```python
from build123d import *

# Parameters (mm, degrees)
BOSS_EXTRUDE1_DEPTH     = 3.5
BOSS_EXTRUDE2_DEPTH     = 7
SKETCH3_R               = 1.5
SKETCH3_W               = 8
SKETCH3_H               = 8
SKETCH3_R_2             = 2.5
BOSS_EXTRUDE3_DEPTH     = 4.5
SKETCH4_R               = 2.5
BOSS_EXTRUDE4_DEPTH     = 4.5
CUT_EXTRUDE1_DEPTH      = 123.693401635
CUT_EXTRUDE1_DEPTH_BACK = 123.693401635
SKETCH5_R               = 2.5
SKETCH5_R_2             = 2.55926668
SKETCH5_R_3             = 1.5
FILLET1_R               = 3.5


with BuildPart() as part:
    # Sketch1 → Boss-Extrude1 (new body)
    with BuildSketch(Plane(origin=(0, 0, 0), x_dir=(1, 0, 0), z_dir=(0, 1, 0))):
        Polygon((-57.597316241, 51.805869074), (-57.597316241, -8.444130926), (-46.097316241, -28.194130926), (-46.097316241, -108.194130926), (43.902683759, -108.194130926), (43.902683759, -28.194130926), (55.402683759, -8.444130926), (55.402683759, 51.805869074), align=None)
    extrude(amount=BOSS_EXTRUDE1_DEPTH)

    # Sketch2 → Boss-Extrude2 (add)
    with BuildSketch(Plane(origin=(0, 3.5, 0), x_dir=(1, 0, 0), z_dir=(0, 1, 0))):
        Polygon((-46.097316241, -28.194130926), (-46.097316241, -108.194130926), (43.902683759, -108.194130926), (43.902683759, -28.194130926), (41.402683759, -28.194130926), (41.402683759, -105.694130926), (-43.597316241, -105.694130926), (-43.597316241, -28.194130926), align=None)
        Polygon((52.902683759, -6.988434723), (55.402683759, -8.444130926), (43.902683759, -28.194130926), (41.402683759, -26.738434723), align=None)
        Polygon((41.402683759, -28.194130926), (43.902683759, -28.194130926), (41.402683759, -26.738434723), align=None)
        Polygon((52.902683759, -6.988434723), (55.402683759, -8.444130926), (55.402683759, -6.988434723), align=None)
        Polygon((-57.597316241, 51.805869074), (-57.597316241, -6.988434723), (-55.097316241, -6.988434723), (-55.097316241, 49.305869074), (52.902683759, 49.305869074), (52.902683759, -6.988434723), (55.402683759, -6.988434723), (55.402683759, 51.805869074), align=None)
        Polygon((-43.597316241, -26.738434723), (-46.097316241, -28.194130926), (-43.597316241, -28.194130926), align=None)
        Polygon((-43.597316241, -26.738434723), (-46.097316241, -28.194130926), (-57.597316241, -8.444130926), (-55.097316241, -6.988434723), align=None)
        Polygon((-57.597316241, -6.988434723), (-57.597316241, -8.444130926), (-55.097316241, -6.988434723), align=None)
    extrude(amount=BOSS_EXTRUDE2_DEPTH)

    # Sketch3 → Boss-Extrude3 (add)
    # profile 1 of 3: a face of its own
    with BuildSketch(Plane(origin=(0, 3.5, 0), x_dir=(1, 0, 0), z_dir=(0, 1, 0))):
        Polygon((-43.597316241, -99.694130926), (-43.597316241, -105.694130926), (41.402683759, -105.694130926), (41.402683759, -99.694130926), (32.902683759, -99.694130926), (20.902683759, -102.694130926), (-23.097316241, -102.694130926), (-35.097316241, -99.694130926), align=None)
        with Locations(Location((-39.347316241, -101.944130926, 0), (0, 0, 270))):
            Circle(SKETCH3_R, mode=Mode.SUBTRACT)
        with Locations(Location((37.152683759, -101.944130926, 0), (0, 0, 270))):
            Circle(SKETCH3_R, mode=Mode.SUBTRACT)
    # profile 2 of 3: a face of its own
    with BuildSketch(Plane(origin=(0, 3.5, 0), x_dir=(1, 0, 0), z_dir=(0, 1, 0))):
        with Locations((-51.097316241, 45.305869074)):
            Rectangle(SKETCH3_W, SKETCH3_H)
        with Locations(Location((-51.097316241, 45.305869074, 0), (0, 0, 270))):
            Circle(SKETCH3_R_2, mode=Mode.SUBTRACT)
    # profile 3 of 3: a face of its own
    with BuildSketch(Plane(origin=(0, 3.5, 0), x_dir=(1, 0, 0), z_dir=(0, 1, 0))):
        with Locations((48.902683759, 45.305869074)):
            Rectangle(SKETCH3_W, SKETCH3_H)
        with Locations(Location((48.902683759, 45.305869074, 0), (0, 0, 270))):
            Circle(SKETCH3_R_2, mode=Mode.SUBTRACT)
    extrude(amount=BOSS_EXTRUDE3_DEPTH)

    # Sketch4 → Boss-Extrude4 (add)
    # profile 1 of 2: a face of its own
    with BuildSketch(Plane(origin=(0, 3.5, 0), x_dir=(1, 0, 0), z_dir=(0, 1, 0))):
        Polygon((1.402683759, 10.130869074), (-55.097316241, 10.130869074), (-55.097316241, -6.988434723), (-43.597316241, -26.738434723), (-43.597316241, 0.130869074), (1.402683759, 0.130869074), align=None)
        with Locations(Location((-31.847316241, 5.130869074, 0), (0, 0, 90))):
            Circle(SKETCH4_R, mode=Mode.SUBTRACT)
        with Locations(Location((-21.847316241, 5.130869074, 0), (0, 0, 90))):
            Circle(SKETCH4_R, mode=Mode.SUBTRACT)
    # profile 2 of 2: a face of its own
    with BuildSketch(Plane(origin=(0, 3.5, 0), x_dir=(1, 0, 0), z_dir=(0, 1, 0))):
        Polygon((39.6145491, 10.130869074), (39.6145491, 0.130869074), (41.402683759, 0.130869074), (41.402683759, -26.738434723), (52.902683759, -6.988434723), (52.902683759, 10.130869074), align=None)
    extrude(amount=BOSS_EXTRUDE4_DEPTH)

    # Sketch5 → Cut-Extrude1 (cut, two sides: drawn at the far end of the back side and taken through both)
    with BuildSketch(Plane(origin=(0, 5, 0), x_dir=(1, 0, 0), z_dir=(0, 1, 0)).offset(-CUT_EXTRUDE1_DEPTH_BACK)):
        with Locations(Location((-21.847316241, 5.130869074, 0), (0, 0, 90))):
            Circle(SKETCH5_R)
        with Locations(Location((-31.847316241, 5.130869074, 0), (0, 0, 270))):
            Circle(SKETCH5_R_2)
        with Locations(Location((-39.347316241, -101.944130926, 0), (0, 0, 270))):
            Circle(SKETCH5_R_3)
        with Locations(Location((37.152683759, -101.944130926, 0), (0, 0, 270))):
            Circle(SKETCH5_R_3)
        with Locations(Location((-51.097316241, 45.305869074, 0), (0, 0, 270))):
            Circle(SKETCH5_R)
        with Locations(Location((48.902683759, 45.305869074, 0), (0, 0, 270))):
            Circle(SKETCH5_R)
        with Locations(Location((-49.597316241, -6.988434723, 0), (0, 0, 270))):
            Circle(SKETCH5_R)
        with Locations(Location((47.402683759, -6.988434723, 0), (0, 0, 270))):
            Circle(SKETCH5_R)
    extrude(amount=CUT_EXTRUDE1_DEPTH + CUT_EXTRUDE1_DEPTH_BACK, mode=Mode.SUBTRACT)

    # Fillet1
    # the kernel refuses this fillet: 3.5 mm, written as the material it adds along each edge
    with BuildSketch(Plane(origin=(41.402683759, 3.5, 99.694130926), x_dir=(0, 0, -1), z_dir=(0, 1, 0)), Plane(origin=(-43.597316241, 3.5, 99.694130926), x_dir=(1, 0, 0), z_dir=(0, 1, 0)), Plane(origin=(-55.097316241, 3.5, -41.305869074), x_dir=(0, 0, 1), z_dir=(0, 1, 0)), Plane(origin=(-47.097316241, 3.5, -49.305869074), x_dir=(0, 0, 1), z_dir=(0, 1, 0)), Plane(origin=(52.902683759, 3.5, -41.305869074), x_dir=(-1, 0, 0), z_dir=(0, 1, 0)), Plane(origin=(-55.097316241, 3.5, -10.130869074), x_dir=(1, 0, 0), z_dir=(0, 1, 0))) as fillet1_piece_1:
        with BuildLine():
            CenterArc((FILLET1_R, FILLET1_R), FILLET1_R, 180, 90)
            Line((0, FILLET1_R), (0, 0))
            Line((0, 0), (FILLET1_R, 0))
        make_face()
    extrude(amount=4.5)
    with BuildSketch(Plane(origin=(20.902683759, 2.422825776, 102.694130926), x_dir=(0.9701425001453338, 0, -0.2425356250363252), z_dir=(0, 1, 0)), Plane(origin=(-23.097316241, 2.422825776, 102.694130926), x_dir=(1, 0, 0), z_dir=(0, 1, 0))) as fillet1_piece_2:
        with BuildLine():
            CenterArc((FILLET1_R * 0.123105625618, FILLET1_R), FILLET1_R, 255.963756532, 14.036243468)
            Line((-FILLET1_R * 0.119429999419, FILLET1_R * 0.0298574998547), (0, 0))
            Line((0, 0), (FILLET1_R * 0.123105625618, 0))
        make_face()
    extrude(amount=5.577174224)
    with BuildSketch(Plane(origin=(44.902683759, 3.5, -49.305869074), x_dir=(0, 0, 1), z_dir=(0, 1, 0)), Plane(origin=(52.902683759, 3.5, -10.130869074), x_dir=(-1, 0, 0), z_dir=(0, 1, 0)), Plane(origin=(-43.597316241, 3.5, -0.130869074), x_dir=(1, 0, 0), z_dir=(0, 1, 0))) as fillet1_piece_3:
        with BuildLine():
            CenterArc((FILLET1_R, -FILLET1_R), FILLET1_R, 90, 90)
            Line((0, -FILLET1_R), (0, 0))
            Line((0, 0), (FILLET1_R, 0))
        make_face()
    extrude(amount=4.5)
    with BuildSketch(Plane(origin=(43.902683759, 10.5, 28.194130926), x_dir=(0, 0, 1), z_dir=(0, -1, 0)), Plane(origin=(-46.097316241, 0, 28.194130926), x_dir=(0, 0, 1), z_dir=(0, 1, 0))) as fillet1_piece_4:
        with BuildLine():
            CenterArc((FILLET1_R * 0.269926710528, -FILLET1_R), FILLET1_R, 90, 30.211322386)
            Line((-FILLET1_R * 0.23326401814, -FILLET1_R * 0.135824618157), (0, 0))
            Line((0, 0), (FILLET1_R * 0.269926710528, 0))
        make_face()
    extrude(amount=10.5)
    with BuildSketch(Plane(origin=(41.402683759, 3.5, -0.130869074), x_dir=(-1, 0, 0), z_dir=(0, 1, 0))) as fillet1_piece_5:
        with BuildLine():
            CenterArc((3.5, 3.052788407), FILLET1_R, 180, 60.718267745)
            Line((0, 3.052788407), (0, 0))
            Line((0, 0), (1.788134659, 0))
        make_face()
    extrude(amount=4.5)
    # the kernel refuses this fillet: 3.5 mm, written as the material it takes off along each edge
    with BuildSketch(Plane(origin=(32.902683759, 3.5, 99.694130926), x_dir=(-0.9701425001453338, 0, 0.2425356250363252), z_dir=(0, 1, 0)), Plane(origin=(-35.097316241, 3.5, 99.694130926), x_dir=(-1, 0, 0), z_dir=(0, 1, 0))) as fillet1_2_piece_1:
        with BuildLine():
            CenterArc((FILLET1_R * 0.123105625618, FILLET1_R), FILLET1_R, 255.963756532, 14.036243468)
            Line((-FILLET1_R * 0.119429999419, FILLET1_R * 0.0298574998547), (0, 0))
            Line((0, 0), (FILLET1_R * 0.123105625618, 0))
        make_face()
    extrude(amount=5.577174224, mode=Mode.SUBTRACT)
    with BuildSketch(Plane(origin=(-47.097316241, 3.5, -41.305869074), x_dir=(0, 0, -1), z_dir=(0, 1, 0)), Plane(origin=(44.902683759, 3.5, -41.305869074), x_dir=(1, 0, 0), z_dir=(0, 1, 0)), Plane(origin=(39.6145491, 3.5, -10.130869074), x_dir=(0, 0, 1), z_dir=(0, 1, 0)), Plane(origin=(1.402683759, 3.5, -10.130869074), x_dir=(-1, 0, 0), z_dir=(0, 1, 0)), Plane(origin=(1.402683759, 3.5, -0.130869074), x_dir=(0, 0, -1), z_dir=(0, 1, 0))) as fillet1_2_piece_2:
        with BuildLine():
            CenterArc((FILLET1_R, FILLET1_R), FILLET1_R, 180, 90)
            Line((0, FILLET1_R), (0, 0))
            Line((0, 0), (FILLET1_R, 0))
        make_face()
    extrude(amount=13.25, mode=Mode.SUBTRACT)
    with BuildSketch(Plane(origin=(55.402683759, 12.861858717, 8.444130926), x_dir=(0, 0, -1), z_dir=(0, -1, 0))) as fillet1_2_piece_3:
        with BuildLine():
            CenterArc((FILLET1_R * 0.269926710528, -FILLET1_R), FILLET1_R, 90, 30.211322386)
            Line((-FILLET1_R * 0.23326401814, -FILLET1_R * 0.135824618157), (0, 0))
            Line((0, 0), (FILLET1_R * 0.269926710528, 0))
        make_face()
    extrude(amount=15.223717434, mode=Mode.SUBTRACT)
    with BuildSketch(Plane(origin=(43.902683759, 19.25, 108.194130926), x_dir=(0, 0, -1), z_dir=(0, -1, 0)), Plane(origin=(55.402683759, -8.75, -51.805869074), x_dir=(0, 0, 1), z_dir=(0, 1, 0))) as fillet1_2_piece_4:
        with BuildLine():
            CenterArc((FILLET1_R, -FILLET1_R), FILLET1_R, 90, 90)
            Line((0, -FILLET1_R), (0, 0))
            Line((0, 0), (FILLET1_R, 0))
        make_face()
    extrude(amount=28, mode=Mode.SUBTRACT)
    with BuildSketch(Plane(origin=(-46.097316241, -8.75, 108.194130926), x_dir=(1, 0, 0), z_dir=(0, 1, 0)), Plane(origin=(-57.597316241, -8.75, -51.805869074), x_dir=(0, 0, 1), z_dir=(0, 1, 0))) as fillet1_2_piece_5:
        with BuildLine():
            CenterArc((FILLET1_R, FILLET1_R), FILLET1_R, 180, 90)
            Line((0, FILLET1_R), (0, 0))
            Line((0, 0), (FILLET1_R, 0))
        make_face()
    extrude(amount=28, mode=Mode.SUBTRACT)
    with BuildSketch(Plane(origin=(-57.597316241, -2.361858717, 8.444130926), x_dir=(0.5031907286678244, 0, 0.8641753818425655), z_dir=(0, 1, 0))) as fillet1_2_piece_6:
        with BuildLine():
            CenterArc((FILLET1_R * 0.269926710528, FILLET1_R), FILLET1_R, 239.788677614, 30.211322386)
            Line((-FILLET1_R * 0.23326401814, FILLET1_R * 0.135824618157), (0, 0))
            Line((0, 0), (FILLET1_R * 0.269926710528, 0))
        make_face()
    extrude(amount=15.223717434, mode=Mode.SUBTRACT)


solid = part.part
```
For this review, take the finished solid that the model builds, in its own axes (mm). A direction names the side the tool comes from. Give positions to 0.01 mm unless a question says otherwise; leave off trailing zeros. Write each loop counter-clockwise with the first axis right and the second up, starting at its lowest first coordinate (ties: lowest second). Pieces come first, ordered by that corner, then holes. Notation, with made-up numbers: M 55.25,46 L 112.25,46 A30 cw 112.25,85 Z; hole C 89.5,50.5 d8. An arc over 180 degrees is marked long. One line per item, written item: value.
1) Take a section at C-C, the plane y = 6. Count the separate pieces of the cut face and the enclosed holes in it, then the cut area to 3 significant figures.
Results are:
separate pieces: 1
enclosed holes: 9
area: 2,740 mm²
2) For line 1 (X direction, y = 8.75, z = -30); line 2 (Z direction, x = -18.5, y = 9.5); line 3 (Y direction, x = -38.5, z = 50), list the stretches that pass through material, from the lowest coordinate up. Write a range as from..to.
Results are:
line 1: x = -57.6..-55.1, 52.9..55.4
line 2: z = -51.81..-49.31, 105.69..108.19
line 3: y = 0..3.5
3) The part is to be moulded in two halves that separate along Z. For faces 3 (the cylindrical face through (-37.86, 3.94, 101.75)), 4 (the flat face through (0, 5, -51.806)), 5 (the cylindrical face through (-42.545, 5.719, 0.867)), 6 (the flat face through (-56, 10.5, -13)), say which applies: +Z half, -Z half, draft (parallel to the pull), parting line (faces both ways), or undercut.
Results are:
face 3: undercut
face 4: -Z half
face 5: undercut
face 6: draft
4) For P1, Ø6, axis at x = -21.85, z = -5.13, coming from the +Y side; P2, Ø1, axis at x = -27, z = 9.5, coming from the +Y side; P3, Ø3, axis at y = 4.5, z = 51.5, coming from the -X side, all flat-tipped, find the tip position at first contact; note any pin that passes through.
Results are:
P1: stops at y = 8
P2: stops at y = 3.5
P3: stops at x = -46.1
5) Take a section at A-A, the plane z = -29.5. Write out the cut boundary in (x, y).
Results are:
outline: M -57.6,0 L 55.4,0 L 55.4,10.5 L 52.9,10.5 L 52.9,3.5 L -55.1,3.5 L -55.1,10.5 L -57.6,10.5 Z
6) For faces 1 (the cylindrical face through (38.64, 3.94, 101.75)), 2 (the cylindrical face through (40.35, 5.719, 98.696)), list the 3-axis set-ups (+Z, -Z, +X, -X, +Y, -Y) from which the entire face can be reached by the end or side of a thin tool; tool diameter is ignored.
Results are:
face 1: +Y, -Y
face 2: +Y
7) Take a section at B-B, the plane x = 16.5. Write out the cut boundary in (y, z), then the cut area to 4 significant figures.
Results are:
outline: M 0,-51.81 L 10.5,-51.81 L 10.5,-49.31 L 3.5,-49.31 L 3.5,102.69 L 8,102.69 L 8,105.69 L 10.5,105.69 L 10.5,108.19 L 0,108.19 Z
area: 608.5 mm²
8) Take a section at D-D, the plane z = 77.5. Write out the cut boundary in (x, y).
Results are:
outline: M -46.1,0 L 43.9,0 L 43.9,10.5 L 41.4,10.5 L 41.4,3.5 L -43.6,3.5 L -43.6,10.5 L -46.1,10.5 Z
